```python
from build123d import *

# Parameters (mm, degrees)
SKETCH1_R           = 12.6365
BOSS_EXTRUDE1_DEPTH = 21.844
SKETCH2_R           = 17.526
BOSS_EXTRUDE2_DEPTH = 3.175
CHAMFER1_SIZE       = 0.254
SKETCH3_R           = 4.09575
CUT_EXTRUDE1_DEPTH  = 34.037579936
CHAMFER2_SIZE       = 0.254


with BuildPart() as part:
    # Sketch1 → Boss-Extrude1 (new body)
    with BuildSketch(Plane(origin=(0, 0, 0), x_dir=(0, 0, -1), z_dir=(1, 0, 0))):
        Circle(SKETCH1_R)
    extrude(amount=BOSS_EXTRUDE1_DEPTH)

    # Sketch2 → Boss-Extrude2 (add)
    with BuildSketch(Plane(origin=(7.9375, 0, 0), x_dir=(0, 0, -1), z_dir=(1, 0, 0))):
        Circle(SKETCH2_R)
    extrude(amount=-BOSS_EXTRUDE2_DEPTH)

    # Chamfer1
    chamfer1_edges = [part.edges().sort_by_distance(p)[0] for p in [
        (0, 0, 12.6365),
        (21.844, 0, 12.6365),
        (4.7625, 0, 12.6365),
        (7.9375, 0, 12.6365),
        (4.7625, 0, 17.526),
        (7.9375, 0, 17.526),
    ]]
    chamfer(chamfer1_edges, length=CHAMFER1_SIZE)

    # Sketch3 → Cut-Extrude1 (cut, through all)
    with BuildSketch(Plane(origin=(21.844, 0, 0), x_dir=(0, 0, -1), z_dir=(1, 0, 0))):
        Circle(SKETCH3_R)
    extrude(amount=-CUT_EXTRUDE1_DEPTH, mode=Mode.SUBTRACT)

    # Chamfer2
    chamfer2_edges = [part.edges().sort_by_distance(p)[0] for p in [
        (0, 0, 4.09575),
        (21.844, 0, 4.09575),
    ]]
    chamfer(chamfer2_edges, length=CHAMFER2_SIZE)


solid = part.part
```
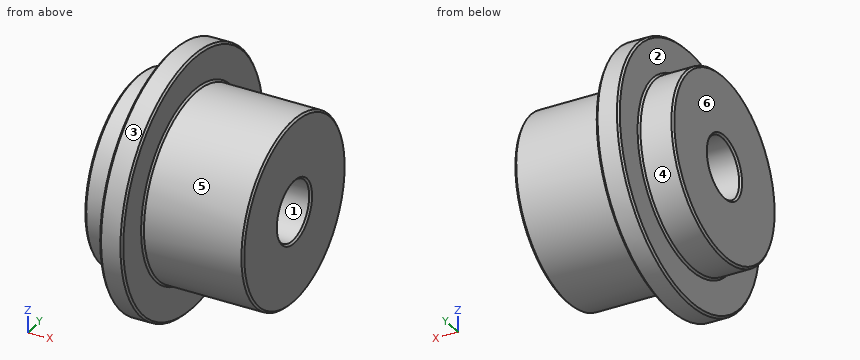
Design review of the part built by this model. Coordinates are the model's own, in mm. Face numbers are marked on the shaded views. A direction names the side the tool comes from. Coordinates: 2 decimals unless noted, no trailing zeros. Order: outer loops, then holes, each group sorted by start corner. A loop starts at its lowest first (then second) coordinate and runs counter-clockwise, first axis right, second up. Notation, with made-up numbers: (15.25, 14.5) - (58.25, 14.5) arc R17 ccw to (58.25, 24.5) - close; hole circle Ø9 at (78.25, 61). An arc over 180 degrees is marked (long way). One line per question, with ' | ' between items.
Q1. For the marked faces 4, 5 and 6, list the 3-axis set-ups (+Z, -Z, +X, -X, +Y, -Y) from which the entire face can be reached by the end or side of a thin tool; tool diameter is ignored.
Answer key:
face 4: -X | face 5: +X | face 6: +Z, -Z, -X, +Y, -Y
Q2. Consider section D-D, the plane x = 19. Give the boundary of the cut face in (y, z).
Answer key:
outline: circle Ø25.27 at (0, 0); hole circle Ø8.19 at (0, 0)
Q3. The part is to be moulded in two halves that separate along Z. For the marked faces 1, 2 and 3, say which applies: +Z half, -Z half, draft (parallel to the pull), parting line (faces both ways), or undercut.
Answer key:
face 1: undercut | face 2: draft | face 3: parting line
Q4. Clearance check with flat-ended pins moving along their axes: pin 1 Ø7.5 at (y, z) = (0, 0) entering from +X; pin 2 Ø2 at (x, z) = (14, -8) entering from +Y; pin 3 Ø12 at (x, z) = (16, 8) entering from +Y; pin 4 Ø3 at (x, y) = (3, 7) entering from +Z. State where each tip first meets the part, or that it passes through.
Answer key:
pin 1: passes through | pin 2: stops at y = 10.52 | pin 3: stops at y = 12.48 | pin 4: stops at z = 11.38
Q5. To check wall thickness, follow line 1 along Y through (x, z) = (14.25, 0); line 2 along Y through (x, z) = (5.25, 0); line 3 along X through (y, z) = (8.5, -13.5). State the ranges of each line that lie inside material, in increasing order.
Answer key:
line 1: y = -12.64 to -4.1, 4.1 to 12.64 | line 2: y = -17.53 to -4.1, 4.1 to 17.53 | line 3: x = 4.76 to 7.94
Q6. Consider section C-C, the plane x = 5.75. Give the boundary of the cut face in (y, z).
Answer key:
outline: circle Ø35.05 at (0, 0); hole circle Ø8.19 at (0, 0)
